```python
from build123d import *

# Parameters (mm, degrees)
BOSS_EXTRUDE1_DEPTH                                 = 2.5
SKETCH1_4_R                                         = 9.75
SKETCH1_4_R_2                                       = 7.75
BOSS_EXTRUDE3_DEPTH                                 = 30
CUT_EXTRUDE1_START                                  = 10
SKETCH1_5_R                                         = 7.75
CUT_EXTRUDE1_DEPTH                                  = 10
CSK_FOR_M3_COUNTERSUNK_FLAT_HEAD_SCREW1_D           = 3.2
CSK_FOR_M3_COUNTERSUNK_FLAT_HEAD_SCREW1_DEPTH       = 2.5
CSK_FOR_M3_COUNTERSUNK_FLAT_HEAD_SCREW1_CSINK_D     = 6.3
CSK_FOR_M3_COUNTERSUNK_FLAT_HEAD_SCREW1_CSINK_ANGLE = 90
CSK_FOR_M3_COUNTERSUNK_FLAT_HEAD_SCREW1_TIP         = 0.96137699


with BuildPart() as part:
    # Sketch1 → Boss-Extrude1 (new body)
    with BuildSketch(Plane(origin=(0, 0, 0), x_dir=(1, 0, 0), z_dir=(0, 1, 0))):
        with BuildLine():
            Line((-37, 60), (-37, -60))
            ThreePointArc((-37, -60), (-34.949747468, -64.949747468), (-30, -67))
            Line((-30, -67), (30, -67))
            ThreePointArc((30, -67), (34.949747468, -64.949747468), (37, -60))
            Line((37, -60), (37, 60))
            ThreePointArc((37, 60), (34.949747468, 64.949747468), (30, 67))
            Line((30, 67), (-30, 67))
            ThreePointArc((-30, 67), (-34.949747468, 64.949747468), (-37, 60))
        make_face()
    extrude(amount=BOSS_EXTRUDE1_DEPTH)

    # Sketch1_4 → Boss-Extrude3 (add)
    with BuildSketch(Plane(origin=(0, 0, 0), x_dir=(1, 0, 0), z_dir=(0, 1, 0))):
        with Locations(Location((0, -27, 0), (0, 0, 270))):
            Circle(SKETCH1_4_R)
        with Locations(Location((0, -27, 0), (0, 0, 270))):
            Circle(SKETCH1_4_R_2, mode=Mode.SUBTRACT)
    extrude(amount=-BOSS_EXTRUDE3_DEPTH)

    # Sketch1_5 → Cut-Extrude1 (cut)
    with BuildSketch(Plane(origin=(0, 0, 0), x_dir=(1, 0, 0), z_dir=(0, 1, 0)).offset(CUT_EXTRUDE1_START)):
        with Locations(Location((0, -27, 0), (0, 0, 270))):
            Circle(SKETCH1_5_R)
    extrude(amount=-CUT_EXTRUDE1_DEPTH, mode=Mode.SUBTRACT)

    # CSK for M3 Countersunk Flat Head Screw1
    with Locations(Plane(origin=(0, 0, 0), x_dir=(-1, 0, 0), z_dir=(0, -1, 0))):
        with Locations((27, -57), (-27, -57), (-27, 57), (27, 57)):
            CounterSinkHole(CSK_FOR_M3_COUNTERSUNK_FLAT_HEAD_SCREW1_D / 2, CSK_FOR_M3_COUNTERSUNK_FLAT_HEAD_SCREW1_CSINK_D / 2, depth=CSK_FOR_M3_COUNTERSUNK_FLAT_HEAD_SCREW1_DEPTH, counter_sink_angle=CSK_FOR_M3_COUNTERSUNK_FLAT_HEAD_SCREW1_CSINK_ANGLE)
            with Locations((0, 0, -(CSK_FOR_M3_COUNTERSUNK_FLAT_HEAD_SCREW1_DEPTH + CSK_FOR_M3_COUNTERSUNK_FLAT_HEAD_SCREW1_TIP / 2))):  # 118° drill point
                Cone(0, CSK_FOR_M3_COUNTERSUNK_FLAT_HEAD_SCREW1_D / 2, CSK_FOR_M3_COUNTERSUNK_FLAT_HEAD_SCREW1_TIP, mode=Mode.SUBTRACT)


solid = part.part
```
Part model, mm, in its own coordinate system. A direction names the side the tool comes from. Give positions to 0.01 mm unless a question says otherwise; leave off trailing zeros. Loops run counter-clockwise (first coordinate to the right, second up) from the corner with the lowest first, then second, coordinate; pieces in that order, holes last. Notation, with made-up numbers: M 78.25,51.25 L 121.25,51.25 A11 ccw 121.25,63.25 Z; hole C 49,54 d4. An arc over 180 degrees is marked long. Return JSON: item names as keys, results as strings.
1) Flat gauge pins, fed straight in: pin 1 Ø5 at (y, z) = (-3, 43.5) entering from -X; pin 2 Ø1 at (x, z) = (-28.5, 39) entering from -Y. Where does each tip first touch, or does it go through?
Calculated:
{"pin 1": "passes through", "pin 2": "stops at y = 0"}
2) Saw through at D-D, the plane y = -18. List the corners of the cut face in (x, z), then the cut area to 3 significant figures.
Calculated:
{"outline": "C 0,27 d19.5; hole C 0,27 d15.5", "area": "110 mm2"}
3) Drill centre lines: line 1 (Z direction, x = -27, y = 2.1); line 2 (X direction, y = -6.5, z = 27); line 3 (Z direction, x = 27, y = 1). Where is each one in solid material? Low to high.
Calculated:
{"line 1": "z = -67 to -58.6, -55.4 to 55.4, 58.6 to 67", "line 2": "x = -9.75 to -7.75, 7.75 to 9.75", "line 3": "z = -67 to -59.15, -54.85 to 54.85, 59.15 to 67"}
4) 3-axis set-ups, long thin cutter, end or side, ignore diameter. For faces 1 (the face through (0, 1, -67)), 2 (the face through (2.93, -14.79, 36.3)): which of +Z, -Z, +X, -X, +Y, -Y reach the whole face in a straight line?
Calculated:
{"face 1": "-Z, +X, -X, +Y, -Y", "face 2": "-Y"}
5) Saw through at C-C, the plane z = 57. List the corners of the cut face in (x, y).
Calculated:
{"outline": "M -37,0 L -30.15,0 L -28.6,1.55 L -28.6,2.5 L -37,2.5 Z; M -25.4,1.55 L -23.85,0 L 23.85,0 L 25.4,1.55 L 25.4,2.5 L -25.4,2.5 Z; M 28.6,1.55 L 30.15,0 L 37,0 L 37,2.5 L 28.6,2.5 Z"}
6) Saw through at A-A, the plane z = 27. List the corners of the cut face in (x, y).
Calculated:
{"outline": "M -37,0 L -9.75,0 L -9.75,-30 L -7.75,-30 L -7.75,2.5 L -37,2.5 Z; M 7.75,-30 L 9.75,-30 L 9.75,0 L 37,0 L 37,2.5 L 7.75,2.5 Z"}
7) Pull direction X, two halves, no side cores. Call faces 3 (the face through (37, 1, 1)), 4 (the face through (-1, 2.5, -1)), 5 (the face through (25.4, 2.03, -57.07)): released by +X, released by -X, zero draft, split by the parting line, or undercut.
Calculated:
{"face 3": "released by +X", "face 4": "zero draft", "face 5": "undercut"}
8) Saw through at B-B, the plane x = -27. List the corners of the cut face in (y, z).
Calculated:
{"outline": "M 0,-67 L 2.5,-67 L 2.5,-58.6 L 1.55,-58.6 L 0,-60.15 Z; M 0,-53.85 L 1.55,-55.4 L 2.5,-55.4 L 2.5,55.4 L 1.55,55.4 L 0,53.85 Z; M 0,60.15 L 1.55,58.6 L 2.5,58.6 L 2.5,67 L 0,67 Z"}
